For this review, take the finished solid that the model builds, in its own axes (mm). A direction names the side the tool comes from. Coordinates: 2 decimals unless noted, no trailing zeros. Loops run counter-clockwise (first coordinate to the right, second up) from the corner with the lowest first, then second, coordinate; pieces in that order, holes last. Notation, with made-up numbers: (1.5, 41) - (49.5, 41) arc R24 ccw to (49.5, 65) - close; hole circle Ø10 at (71, 61.5). An arc over 180 degrees is marked (long way). Answer as a JSON object with one key per item and string values. Group by question number.
Item 1: We need section D-D (y = 2.5). Give the boundary of the cut face in (x, z), then the cut area to 3 significant figures.
Item 2: Clearance check with flat-ended pins moving along their axes: pin 1 (1.6 mm diameter, centred on x = 2.5, y = 2.5, fed in from +Z); pin 2 (0.6 mm diameter, centred on x = 11.5, z = 1, fed in from -Y); pin 3 (3 mm diameter, centred on x = 1, z = 12, fed in from -Y); pin 4 (0.6 mm diameter, centred on x = 11.5, z = 1, fed in from +Y). State where each tip first meets the part, or that it passes through.
Item 3: We need section B-B (z = 15.5). Give the boundary of the cut face in (x, y), then the cut area to 3 significant figures.
Item 4: To check wall thickness, follow line 1 (Y direction, x = 2.5, z = 0.55); line 2 (X direction, y = 10.25, z = 12.75); line 3 (Z direction, x = 9, y = 11.25). State the ranges of each line that lie inside material, in increasing order.
Item 5: We need section C-C (y = 12.5). Give the boundary of the cut face in (x, z).
Item 6: Tool access review of faces 5 (the flat face through (1, 15, 12)), 6 (the flat face through (1, 10, 12)), 7 (the flat face through (5, 3, 1)): name each direction out of +Z, -Z, +X, -X, +Y, -Y from which nothing blocks a thin tool from reaching the whole face with its end or side.
Item 7: We need section A-A (y = 8.25). Give the boundary of the cut face in (x, z), then the cut area to 3 significant figures.
Item 8: Mouldability with a two-part tool opening along X and no side actions: class faces 1 (the flat face through (24, 13, 18)), 2 (the flat face through (2.75, 12, 8)), 3 (the flat face through (22.25, 12, 8)), 4 (the flat face through (0, 12, 6)) as released by +X, released by -X, zero draft, split by the parting line, or undercut.
from build123d import *

# Parameters (mm, degrees)
SKETCH_W        = 25
SKETCH_H        = 25
SKETCH_R        = 1
PAD_DEPTH       = 2
SKETCH001_W     = 2.75
SKETCH001_H     = 15
PAD001_DEPTH    = 16
SKETCH002_W     = 15
SKETCH002_H     = 8.75
POCKET_DEPTH    = 100
CHAMFER_SIZE    = 2
SKETCH003_R     = 1
POCKET001_DEPTH = 100
POCKET002_DEPTH = 100


with BuildPart() as part:
    # Sketch → Pad (new body)
    with BuildSketch(Plane.XY):
        with Locations((12.5, 12.5)):
            Rectangle(SKETCH_W, SKETCH_H)
        with Locations((2.5, 22.5)):
            Circle(SKETCH_R, mode=Mode.SUBTRACT)
        with Locations((22.5, 22.5)):
            Circle(SKETCH_R, mode=Mode.SUBTRACT)
        with Locations((22.5, 2.5)):
            Circle(SKETCH_R, mode=Mode.SUBTRACT)
        with Locations((2.5, 2.5)):
            Circle(SKETCH_R, mode=Mode.SUBTRACT)
    extrude(amount=PAD_DEPTH)

    # Sketch001 (on Face10 of Pad) → Pad001 (join)
    with BuildSketch(Plane.XY.offset(2)):
        with Locations((1.375, 12.5)):
            Rectangle(SKETCH001_W, SKETCH001_H)
        with Locations((23.625, 12.5)):
            Rectangle(SKETCH001_W, SKETCH001_H)
    extrude(amount=PAD001_DEPTH)

    # Sketch002 (on Face5 of Pad001) → Pocket (cut)
    with BuildSketch(Plane.XY.offset(2)):
        with Locations((12.5, 20.625)):
            Rectangle(SKETCH002_W, SKETCH002_H)
        with Locations((12.5, 4.375)):
            Rectangle(SKETCH002_W, SKETCH002_H)
    extrude(amount=-POCKET_DEPTH, mode=Mode.SUBTRACT)

    # Chamfer
    chamfer_edges = [part.edges().sort_by_distance(p)[0] for p in [
        (20, 16.25, 1),
        (5, 16.25, 1),
        (5, 8.75, 1),
        (20, 8.75, 1),
    ]]
    chamfer(chamfer_edges, length=CHAMFER_SIZE)

    # Sketch003 (on Face24 of Chamfer) → Pocket001 (cut)
    with BuildSketch(Plane.YZ.offset(25)):
        with Locations((12.5, 15.5)):
            Circle(SKETCH003_R)
    extrude(amount=-POCKET001_DEPTH, mode=Mode.SUBTRACT)

    # Sketch004 (on Face24 of Pocket001) → Pocket002 (cut)
    with BuildSketch(Plane.YZ.offset(25)):
        Polygon((10, 18), (10, 6), (5, 2), (5, 18), align=None)
        Polygon((15, 18), (15, 6), (20, 2), (20, 18), align=None)
    extrude(amount=-POCKET002_DEPTH, mode=Mode.SUBTRACT)


solid = part.part
Check sheet entries:
{
 "1": {"outline": "(0, 0) - (1.5, 0) - (1.5, 2) - (0, 2) - close; (3.5, 0) - (5, 0) - (5, 2) - (3.5, 2) - close; (20, 0) - (21.5, 0) - (21.5, 2) - (20, 2) - close; (23.5, 0) - (25, 0) - (25, 2) - (23.5, 2) - close", "area": "12.0 mm2"},
 "2": {"pin 1": "passes through", "pin 2": "stops at y = 8.75", "pin 3": "stops at y = 10", "pin 4": "stops at y = 16.25"},
 "3": {"outline": "(0, 10) - (2.75, 10) - (2.75, 11.5) - (0, 11.5) - close; (0, 13.5) - (2.75, 13.5) - (2.75, 15) - (0, 15) - close; (22.25, 10) - (25, 10) - (25, 11.5) - (22.25, 11.5) - close; (22.25, 13.5) - (25, 13.5) - (25, 15) - (22.25, 15) - close", "area": "16.5 mm2"},
 "4": {"line 1": "y = 0 to 1.5, 3.5 to 21.5, 23.5 to 25", "line 2": "x = 0 to 2.75, 22.25 to 25", "line 3": "z = 0 to 2"},
 "5": {"outline": "(0, 0) - (25, 0) - (25, 14.5) - (22.25, 14.5) - (22.25, 2) - (2.75, 2) - (2.75, 14.5) - (0, 14.5) - close; (0, 16.5) - (2.75, 16.5) - (2.75, 18) - (0, 18) - close; (22.25, 16.5) - (25, 16.5) - (25, 18) - (22.25, 18) - close"},
 "6": {"face 5": "+Z, +X, -X, +Y", "face 6": "+Z, +X, -X, -Y", "face 7": "+Z, -Z, -Y"},
 "7": {"outline": "(0, 0) - (6.5, 0) - (6.5, 2) - (2.75, 2) - (2.75, 4.6) - (0, 4.6) - close; (18.5, 0) - (25, 0) - (25, 4.6) - (22.25, 4.6) - (22.25, 2) - (18.5, 2) - close", "area": "40.3 mm2"},
 "8": {"face 1": "zero draft", "face 2": "undercut", "face 3": "undercut", "face 4": "released by -X"}
}
